The figure shows three views and two pictorial views of one solid part (mm, origin at its lowest corner). Answer the questions. Round coordinates to 2 decimals unless told otherwise and drop trailing zeros. Return JSON: item names as keys, results as strings. Group by question number.
(1) This flat-tipped pin is pushed along its axis until it touches: pin 1 (4.5 mm diameter, centred on x = 12.7, y = 19.05, fed in from +Z). Where does it stop, or does it pass through?
(2) The part is cut by section A-A (z = 2.65). Count the separate pieces of the cut face and the enclosed holes in it.
(3) Consider line 1 (Y direction, x = 298.45, z = 0.7) (1 decimal); line 2 (X direction, y = 6.75, z = 2.8); line 3 (X direction, y = 20, z = 0.8). Determine where each line is inside the solid, lowest interval first. Write a range as [from, to].
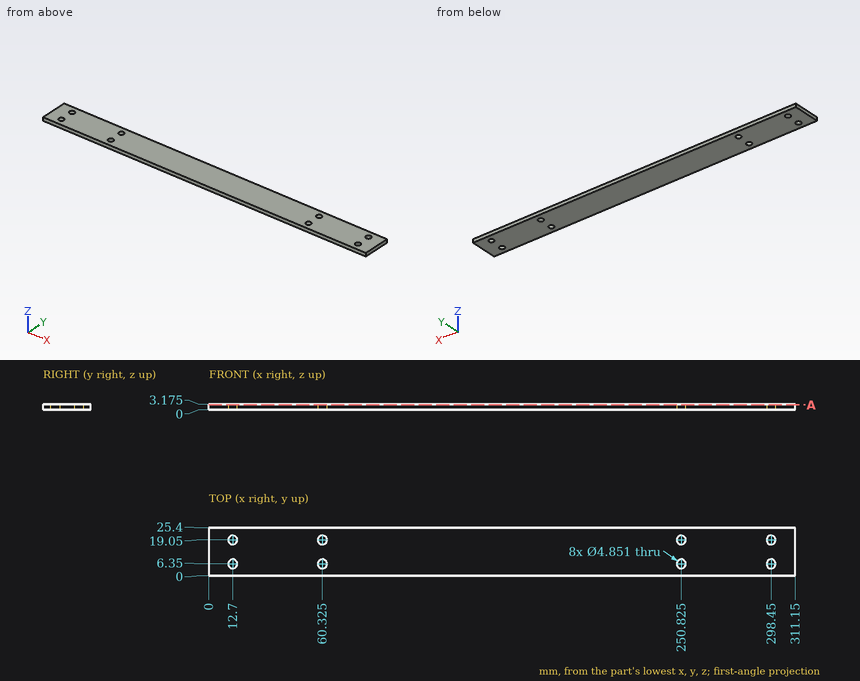
Answer below:
{
 "1": {"pin 1": "passes through"},
 "2": {"separate pieces": "1", "enclosed holes": "8"},
 "3": {"line 1": "y = [0, 3.9], [8.8, 16.6], [21.5, 25.4]", "line 2": "x = [0, 10.31], [15.09, 57.93], [62.72, 248.43], [253.22, 296.06], [300.84, 311.15]", "line 3": "x = [0, 10.47], [14.93, 58.09], [62.56, 248.59], [253.06, 296.22], [300.68, 311.15]"}
}
